```python
from build123d import *

# Parameters (mm, degrees)
SKETCH1_R                = 10
BOSS_EXTRUDE1_DEPTH      = 200
BOSS_EXTRUDE2_DEPTH      = 15
BOSS_EXTRUDE2_DEPTH_BACK = 15
SKETCH2_W                = 125
SKETCH2_H                = 20
BOSS_EXTRUDE3_DEPTH      = 10
BOSS_EXTRUDE3_DEPTH_BACK = 10
SKETCH3_W                = 25
SKETCH3_H                = 75
BOSS_EXTRUDE4_DEPTH      = 5
BOSS_EXTRUDE4_DEPTH_BACK = 5
SKETCH5_W                = 26.648824617
SKETCH5_H                = 125
BOSS_EXTRUDE5_DEPTH      = 5
BOSS_EXTRUDE5_DEPTH_BACK = 5
SKETCH6_RX               = 23.77956847
SKETCH6_RY               = 14.659300575
FILLET1_R                = 10
FILLET2_R                = 10
SKETCH7_RX               = 22.5
SKETCH7_RY               = 13.75
CUT_EXTRUDE1_DEPTH       = 7.5
FILLET3_R                = 5


with BuildPart() as part:
    # Sketch1 → Boss-Extrude1 (new body)
    with BuildSketch(Plane(origin=(0, 0, 0), x_dir=(1, 0, 0), z_dir=(0, 1, 0))):
        with Locations(Location((0, 0, 0), (0, 0, 270))):
            Circle(SKETCH1_R)
    extrude(amount=BOSS_EXTRUDE1_DEPTH)

    # Sketch2 → Boss-Extrude2 (add, two sides: drawn at the far end of the back side and taken through both)
    with BuildSketch(Plane(origin=(0, 0, 0), x_dir=(0, 0, -1), z_dir=(1, 0, 0)).offset(-BOSS_EXTRUDE2_DEPTH_BACK)):
        with Locations((0, 210)):
            Rectangle(SKETCH2_W, SKETCH2_H)
    extrude(amount=BOSS_EXTRUDE2_DEPTH + BOSS_EXTRUDE2_DEPTH_BACK)

    # Sketch3 → Boss-Extrude3 (add, two sides: drawn at the far end of the back side and taken through both)
    with BuildSketch(Plane(origin=(0, 0, 0), x_dir=(0, 0, -1), z_dir=(1, 0, 0)).offset(-BOSS_EXTRUDE3_DEPTH_BACK)):
        with Locations((-25, 257.5)):
            Rectangle(SKETCH3_W, SKETCH3_H)
        with Locations((26.648824617, 257.5)):
            Rectangle(SKETCH3_W, SKETCH3_H)
    extrude(amount=BOSS_EXTRUDE3_DEPTH + BOSS_EXTRUDE3_DEPTH_BACK)

    # Sketch5 → Boss-Extrude4 (add, two sides: drawn at the far end of the back side and taken through both)
    with BuildSketch(Plane(origin=(0, 0, 0), x_dir=(0, 0, -1), z_dir=(1, 0, 0)).offset(-BOSS_EXTRUDE4_DEPTH_BACK)):
        with Locations((0.824412309, 320)):
            Rectangle(SKETCH5_W, SKETCH5_H)
    extrude(amount=BOSS_EXTRUDE4_DEPTH + BOSS_EXTRUDE4_DEPTH_BACK)

    # Sketch6 → Boss-Extrude5 (add, two sides: drawn at the far end of the back side and taken through both)
    with BuildSketch(Plane(origin=(0, 0, 0), x_dir=(0, 0, -1), z_dir=(1, 0, 0)).offset(-BOSS_EXTRUDE5_DEPTH_BACK)):
        with Locations(Location((0.824412308, 402.5), (0, 0, -90))):
            Ellipse(SKETCH6_RX, SKETCH6_RY)
    extrude(amount=BOSS_EXTRUDE5_DEPTH + BOSS_EXTRUDE5_DEPTH_BACK)

    # Fillet1
    # the kernel refuses this fillet: 10 mm, written as the material it takes off along each edge
    with BuildSketch(Plane(origin=(-27.190897542, 382.5, -14.148824617), x_dir=(0, 0, 1), z_dir=(1, 0, 0))) as fillet1_piece_1:
        with BuildLine():
            CenterArc((10, 8.876359017), FILLET1_R, 180, 62.577662354)
            Line((0, 8.876359017), (0, 0))
            Line((0, 0), (5.394541216, 0))
        make_face()
    extrude(amount=27.190898125, mode=Mode.SUBTRACT)
    with BuildSketch(Plane(origin=(5.84e-07, 382.5, -14.148824617), x_dir=(0, 0, 1), z_dir=(1, 0, 0))) as fillet1_piece_2:
        with BuildLine():
            CenterArc((10, 8.876359017), FILLET1_R, 180, 62.577662354)
            Line((0, 8.876359017), (0, 0))
            Line((0, 0), (5.394541216, 0))
        make_face()
    extrude(amount=27.190896958, mode=Mode.SUBTRACT)

    # Fillet2
    # the kernel refuses this fillet: 10 mm, written as the material it takes off along each edge
    with BuildSketch(Plane(origin=(27.190897542, 382.5, 12.5), x_dir=(0, 0, -1), z_dir=(-1, 0, 0))) as fillet2_piece_1:
        with BuildLine():
            CenterArc((10, 8.876359017), FILLET2_R, 180, 62.577662355)
            Line((0, 8.876359017), (0, 0))
            Line((0, 0), (5.394541216, 0))
        make_face()
    extrude(amount=27.190896946, mode=Mode.SUBTRACT)
    with BuildSketch(Plane(origin=(5.96e-07, 382.5, 12.5), x_dir=(0, 0, -1), z_dir=(-1, 0, 0))) as fillet2_piece_2:
        with BuildLine():
            CenterArc((10, 8.876359017), FILLET2_R, 180, 62.577662354)
            Line((0, 8.876359017), (0, 0))
            Line((0, 0), (5.394541216, 0))
        make_face()
    extrude(amount=27.190898138, mode=Mode.SUBTRACT)

    # Sketch7 → Cut-Extrude1 (cut)
    with BuildSketch(Plane(origin=(5, 0, 0), x_dir=(0, 0, -1), z_dir=(1, 0, 0))):
        with Locations(Location((0.824412308, 402.5), (0, 0, 90))):
            Ellipse(SKETCH7_RX, SKETCH7_RY)
    extrude(amount=-CUT_EXTRUDE1_DEPTH, mode=Mode.SUBTRACT)

    # Fillet3
    fillet3_edges = [part.edges().sort_by_distance(p)[0] for p in [
        (-2.5, 380.000046084, -0.852241692),
    ]]
    fillet(fillet3_edges, radius=FILLET3_R)


solid = part.part
```
Here's how the part is built. I have some questions about the finished solid (model axes, mm). A direction names the side the tool comes from. Round coordinates to 2 decimals unless told otherwise and drop trailing zeros. Order: outer loops, then holes, each group sorted by start corner. A loop starts at its lowest first (then second) coordinate and runs counter-clockwise, first axis right, second up. Notation, with made-up numbers: M 10.5,41 L 30.5,41 A18 ccw 30.5,66 Z; hole C -24,20.25 d2. An arc over 180 degrees is marked long. Use CSV: the item, a comma, the result in double quotes.
1) I'm going to push flat-ended pins straight in: P1, Ø20, axis at y = 269.5, z = 25.5, coming from the -X side; P2, Ø10, axis at x = 8, y = 69, coming from the +Z side; P3, Ø1.5, axis at x = -2, z = -24, coming from the -Y side; P4, Ø11, axis at x = 1, z = -6.5, coming from the -Y side. Where does each tip first touch, or does it pass through?
Taken from the geometry:
P1,"x = -10"
P2,"z = 9.54"
P3,"y = 200"
P4,"y = 0"
2) I need wall thicknesses on line 1 along Z through (x, y) = (-9.25, 272); line 2 along Z through (x, y) = (-0.75, 55.5); line 3 along Y through (x, z) = (5, -37.5). Which ranges of each line are inside material? Lowest first, please. Write a range as [from, to].
Taken from the geometry:
line 1,"[-39.15, -14.15], [12.5, 37.5]"
line 2,"[-9.97, 9.97]"
line 3,"[200, 295]"
3) I want a section at B-B (y = 47.5). List the corners of the cut face in (x, z) for me.
Taken from the geometry:
outline,"C 0,0 d20"
4) If we mould it in two halves opening along Z, with no side actions, what happens to faces 1 (the flat face through (0, 334, -14.149)), 2 (the flat face through (-10, 258, -26)), 3 (the flat face through (0, 249, 12.5))? For each: pulls with the +Z half, pulls with the -Z half, needs draft (parallel to the pull), parting line crosses it, or undercut.
Taken from the geometry:
face 1,"pulls with the -Z half"
face 2,"needs draft"
face 3,"undercut"
5) I want a section at A-A (z = -31). List the corners of the cut face in (x, y) for me.
Taken from the geometry:
outline,"M -15,200 L 15,200 L 15,220 L 10,220 L 10,295 L -10,295 L -10,220 L -15,220 Z"
6) On a 3-axis mill with a long thin cutter (end or side, diameter ignored), from which of +Z, -Z, +X, -X, +Y, -Y can I reach the whole of each face in a straight line? I mean faces 4 (the flat face through (10, 258, 25)), 5 (the flat face through (-2.5, 402, -1)), 6 (the flat face through (0, 257, -39.149)), 7 (the flat face through (5, 324, -1)), 8 (the flat face through (0, 249, -14.149)). Say none if no direction works.
Taken from the geometry:
face 4,"+Z, -Z, +X, +Y"
face 5,"+X"
face 6,"-Z, +X, -X, +Y"
face 7,"+X, +Y"
face 8,"none"
